Model file for the job. Use its own axes, mm. Face numbers are marked on the shaded views. A direction names the side the tool comes from. Coordinates: 2 decimals unless noted, no trailing zeros. Write each loop counter-clockwise with the first axis right and the second up, starting at its lowest first coordinate (ties: lowest second). Pieces come first, ordered by that corner, then holes.
Q1. Which spindle directions (+Z, -Z, +X, -X, +Y, -Y) get a long thin tool onto all of the face, cutting with end or side? Do the marked faces 4 and 5. Say none if no direction does.
Q2. Pull direction X, two halves, no side cores. Call the marked faces 1, 2 and 3: released by +X, released by -X, zero draft, split by the parting line, or undercut.
Q3. Band-saw the part on C-C, the plane z = 31.75. State how many separate pieces and enclosed holes the cut face has, plus the area to 3 significant figures.
Q4. Drill centre lines: probe 1 along X at (y, z) = (-2, 32.25); probe 2 along Y at (x, z) = (27, 33). Where is each one in solid material? Low to high.
Q5. Band-saw the part on B-B, the plane y = -16.5. Write the cut outline in (x, z), plus the area to 3 significant figures.
Q6. Pin check, flat tips, straight feed: P1, Ø0.9, axis at x = -25.5, y = -0.5, coming from the +Z side; P2, Ø4, axis at x = 15.5, z = 32.5, coming from the +Y side; P3, Ø1, axis at x = -25.5, z = 31, coming from the +Y side. Stop position of each tip, or through.
Q7. Band-saw the part on A-A, the plane x = 26. Write the cut outline in (y, z).
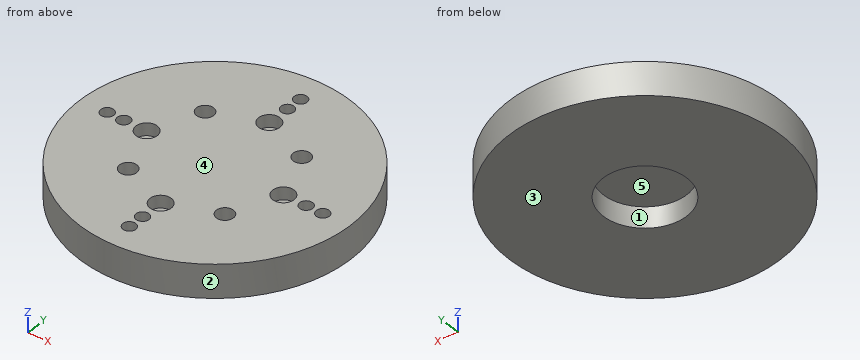
from build123d import *

# Parameters (mm, degrees)
SKETCH1_R           = 55
BOSS_EXTRUDE1_DEPTH = 26
SKETCH2_R           = 1.5
CUT_EXTRUDE1_DEPTH  = 3
SKETCH3_R           = 32.5
BOSS_EXTRUDE2_DEPTH = 8
SKETCH4_R           = 2.55
SKETCH4_R_2         = 1.55
SKETCH4_R_3         = 2.05
CUT_EXTRUDE2_DEPTH  = 3
FILLET1_R           = 2
SKETCH9_R           = 75
CUT_EXTRUDE5_DEPTH  = 83.012194282
SKETCH11_R          = 10
CUT_EXTRUDE6_DEPTH  = 5


with BuildPart() as part:
    # Sketch1 → Boss-Extrude1 (new body)
    with BuildSketch(Plane.XY):
        with Locations(Location((0, 0, 0), (0, 0, 180))):
            Circle(SKETCH1_R)
    extrude(amount=BOSS_EXTRUDE1_DEPTH)

    # Sketch2 → Cut-Extrude1 (cut)
    with BuildSketch(Plane(origin=(0, 0, 0), x_dir=(-1, 0, 0), z_dir=(0, 0, -1))):
        with Locations((0, -21)):
            Circle(SKETCH2_R)
        with Locations((-14.849242405, -14.849242405)):
            Circle(SKETCH2_R)
        with Locations((-21, 0)):
            Circle(SKETCH2_R)
        with Locations((-14.849242405, 14.849242405)):
            Circle(SKETCH2_R)
        with Locations((0, 21)):
            Circle(SKETCH2_R)
        with Locations((14.849242405, 14.849242405)):
            Circle(SKETCH2_R)
        with Locations((21, 0)):
            Circle(SKETCH2_R)
        with Locations((14.849242405, -14.849242405)):
            Circle(SKETCH2_R)
    extrude(amount=-CUT_EXTRUDE1_DEPTH, mode=Mode.SUBTRACT)

    # Sketch3 → Boss-Extrude2 (add)
    with BuildSketch(Plane.XY.offset(26)):
        Circle(SKETCH3_R)
    extrude(amount=BOSS_EXTRUDE2_DEPTH)

    # Sketch4 → Cut-Extrude2 (cut)
    with BuildSketch(Plane.XY.offset(34)):
        with Locations((-16.5, 0)):
            Circle(SKETCH4_R)
        with Locations((0, -16.5)):
            Circle(SKETCH4_R)
        with Locations((16.5, 0)):
            Circle(SKETCH4_R)
        with Locations((0, 16.5)):
            Circle(SKETCH4_R)
        with Locations((0, 26)):
            Circle(SKETCH4_R_2)
        with Locations((0, 22)):
            Circle(SKETCH4_R_2)
        with Locations((-11.66726189, -11.66726189)):
            Circle(SKETCH4_R_3)
        with Locations((11.66726189, -11.66726189)):
            Circle(SKETCH4_R_3)
        with Locations((11.66726189, 11.66726189)):
            Circle(SKETCH4_R_3)
        with Locations((-11.66726189, 11.66726189)):
            Circle(SKETCH4_R_3)
        with Locations((-22, 0)):
            Circle(SKETCH4_R_2)
        with Locations((-26, 0)):
            Circle(SKETCH4_R_2)
        with Locations((0, -22)):
            Circle(SKETCH4_R_2)
        with Locations((0, -26)):
            Circle(SKETCH4_R_2)
        with Locations((22, 0)):
            Circle(SKETCH4_R_2)
        with Locations((26, 0)):
            Circle(SKETCH4_R_2)
    extrude(amount=-CUT_EXTRUDE2_DEPTH, mode=Mode.SUBTRACT)

    # Fillet1
    fillet1_edges = [part.edges().sort_by_distance(p)[0] for p in [
        (55, 0, 0),
        (55, 0, 26),
    ]]
    fillet(fillet1_edges, radius=FILLET1_R)

    # Sketch9 → Cut-Extrude5 (cut, through all)
    with BuildSketch(Plane.XY.offset(26)):
        Circle(SKETCH9_R)
    extrude(amount=-CUT_EXTRUDE5_DEPTH, mode=Mode.SUBTRACT)

    # Sketch11 → Cut-Extrude6 (cut)
    with BuildSketch(Plane(origin=(0, 0, 26), x_dir=(-1, 0, 0), z_dir=(0, 0, -1))):
        Circle(SKETCH11_R)
    extrude(amount=-CUT_EXTRUDE6_DEPTH, mode=Mode.SUBTRACT)


solid = part.part
Answer sheet:
1. face 4: +Z, +X, -X, +Y, -Y
1. face 5: -Z
2. face 1: undercut
2. face 2: split by the parting line
2. face 3: zero draft
3. separate pieces: 1
3. enclosed holes: 16
3. area: 3,120 mm2
4. probe 1: x = -32.44 to -18.08, -14.92 to 14.92, 18.08 to 32.44
4. probe 2: y = -18.09 to -1.18, 1.18 to 18.09
5. outline: (-28, 26) - (28, 26) - (28, 34) - (2.55, 34) - (2.55, 31) - (-2.55, 31) - (-2.55, 34) - (-28, 34) - close
5. area: 433 mm2
6. P1: stops at z = 31
6. P2: stops at y = 29.56
6. P3: stops at y = 20.77
7. outline: (-19.5, 26) - (19.5, 26) - (19.5, 34) - (1.55, 34) - (1.55, 31) - (-1.55, 31) - (-1.55, 34) - (-19.5, 34) - close
